Could you check a few things on this model? Use its own coordinates, in mm. A direction names the side the tool comes from. Round coordinates to 2 decimals unless told otherwise and drop trailing zeros. Write each loop counter-clockwise with the first axis right and the second up, starting at its lowest first coordinate (ties: lowest second). Pieces come first, ordered by that corner, then holes. Notation, with made-up numbers: M 76.5,35.5 L 109.5,35.5 A29 ccw 109.5,60.5 Z; hole C 26.25,45 d1. An arc over 180 degrees is marked long. One line per item, written item: value. Start each with the question number.
(1) Thinking about a two-plate mould opening in X: for faces 1 (the face through (-1.87, -1.55, 0.34)), 2 (the face through (22.68, 0.446, 1.417)), 3 (the face through (24.105, 0, 0)), 4 (the face through (19.2, 0.446, -1.417)), which applies, released by +X, released by -X, zero draft, split by the parting line, or undercut?
(2) I want a section at A-A on x = -2.25. Please give me the cut outline in (y, z) (1 decimal).
(3) If I drill on L1, parallel to X at y = 1.25, z = -0.9; L2, parallel to Y at x = 9, z = 0.55; L3, parallel to Z at x = 9.25, y = 0.35, over which ranges is the centre line in solid material (lowest first)?
(4) Which directions (+Z, -Z, +X, -X, +Y, -Y) give clear straight access to the entire face, cutting with the end or side of a thin tool? Please do faces 5 (the face through (20.96, -1.55, 0.34)), 6 (the face through (-3.63, 0.446, -1.417)).
```python
from build123d import *

# Parameters (mm, degrees)
SKETCH2_R               = 1.5875
EXTRUDE1_DEPTH          = 25.4
EXTRUDE1_DEPTH_BACK     = 25.4
CHAMFER1_SIZE           = 0.3175
SKETCH3_OUTSIDE_W       = 15.376
SKETCH3_OUTSIDE_H       = 15.376
SKETCH3_OUTSIDE_R       = 1.4859
CUT_EXTRUDE1_DEPTH      = 0.3048
SKETCH4_OUTSIDE_W       = 15.376
SKETCH4_OUTSIDE_H       = 15.376
SKETCH4_OUTSIDE_R       = 1.4859
CUT_EXTRUDE2_DEPTH      = 0.3048
CUT_EXTRUDE4_START      = -3.175
SKETCH6_OUTSIDE_W       = 15.376
SKETCH6_OUTSIDE_H       = 15.376
SKETCH6_OUTSIDE_R       = 1.4859
CUT_EXTRUDE4_DEPTH      = 0.3048
CUT_EXTRUDE5_START      = -3.175
SKETCH8_OUTSIDE_W       = 15.376
SKETCH8_OUTSIDE_H       = 15.376
SKETCH8_OUTSIDE_R       = 1.4859
CUT_EXTRUDE5_DEPTH      = 0.3048
SKETCH5_W               = 20.3454
SKETCH5_H               = 6.35
SKETCH5_W_2             = 1.2954
CUT_EXTRUDE3_DEPTH      = 2.5875
CUT_EXTRUDE3_DEPTH_BACK = 2.5875


with BuildPart() as part:
    # Sketch2 → Extrude1 (new body, two sides)
    with BuildSketch(Plane(origin=(0, 0, 0), x_dir=(0, 0, -1), z_dir=(1, 0, 0))) as extrude1_sk:
        Circle(SKETCH2_R)
    extrude(amount=EXTRUDE1_DEPTH)
    extrude(extrude1_sk.sketch, amount=-EXTRUDE1_DEPTH_BACK)

    # Chamfer1
    chamfer1_edges = [part.edges().sort_by_distance(p)[0] for p in [
        (-25.4, 0, 1.5875),
        (25.4, 0, 1.5875),
    ]]
    chamfer(chamfer1_edges, length=CHAMFER1_SIZE)

    # Sketch3 outside → Cut-Extrude1 (cut)
    with BuildSketch(Plane(origin=(19.05, 0, 0), x_dir=(0, 0, -1), z_dir=(1, 0, 0))):
        Rectangle(SKETCH3_OUTSIDE_W, SKETCH3_OUTSIDE_H)
        Circle(SKETCH3_OUTSIDE_R, mode=Mode.SUBTRACT)
    extrude(amount=CUT_EXTRUDE1_DEPTH, mode=Mode.SUBTRACT)

    # Sketch4 outside → Cut-Extrude2 (cut)
    with BuildSketch(Plane(origin=(0, 0, 0), x_dir=(0, 0, -1), z_dir=(1, 0, 0))):
        Rectangle(SKETCH4_OUTSIDE_W, SKETCH4_OUTSIDE_H)
        Circle(SKETCH4_OUTSIDE_R, mode=Mode.SUBTRACT)
    extrude(amount=-CUT_EXTRUDE2_DEPTH, mode=Mode.SUBTRACT)

    # Sketch6 outside → Cut-Extrude4 (cut)
    with BuildSketch(Plane.ZY.offset(-19.3548).offset(CUT_EXTRUDE4_START)):
        Rectangle(SKETCH6_OUTSIDE_W, SKETCH6_OUTSIDE_H)
        Circle(SKETCH6_OUTSIDE_R, mode=Mode.SUBTRACT)
    extrude(amount=-CUT_EXTRUDE4_DEPTH, mode=Mode.SUBTRACT)

    # Sketch8 outside → Cut-Extrude5 (cut)
    with BuildSketch(Plane(origin=(-0.3048, 0, 0), x_dir=(0, 0, -1), z_dir=(1, 0, 0)).offset(CUT_EXTRUDE5_START)):
        Rectangle(SKETCH8_OUTSIDE_W, SKETCH8_OUTSIDE_H)
        Circle(SKETCH8_OUTSIDE_R, mode=Mode.SUBTRACT)
    extrude(amount=-CUT_EXTRUDE5_DEPTH, mode=Mode.SUBTRACT)

    # Sketch5 → Cut-Extrude3 (cut, two sides)
    with BuildSketch(Plane.XY) as cut_extrude3_sk:
        with Locations((-15.2273, 0)):
            Rectangle(SKETCH5_W, SKETCH5_H)
        with Locations((24.7523, 0)):
            Rectangle(SKETCH5_W_2, SKETCH5_H)
    extrude(amount=CUT_EXTRUDE3_DEPTH, mode=Mode.SUBTRACT)
    extrude(cut_extrude3_sk.sketch, amount=-CUT_EXTRUDE3_DEPTH_BACK, mode=Mode.SUBTRACT)


solid = part.part
```
Found:
1. face 1: zero draft
1. face 2: undercut
1. face 3: released by +X
1. face 4: undercut
2. outline: C 0,0 d3.2
3. L1: x = -5.05 to -3.78, -3.48 to -0.3, 0 to 19.05, 19.35 to 22.53, 22.83 to 24.1
3. L2: y = -1.49 to 1.49
3. L3: z = -1.55 to 1.55
4. face 5: +X, -X
4. face 6: none
